```python
from build123d import *

# Parameters (mm, degrees)
SKETCH9_OUTSIDE_W          = 164.226
SKETCH9_OUTSIDE_H          = 164.226
BODY_CUT_DEPTH             = 177.452945975
SKETCH10_OUTSIDE_W         = 127.798
SKETCH10_OUTSIDE_H         = 127.798
BODY_CUT_INNER_DEPTH       = 76.981920155
CUT_FIXING_HOLE_START      = -39.50904
SKETCH15_R                 = 2.75
CUT_FIXING_HOLE_DEPTH      = 39.50904
SKETCH16_R                 = 1.25
CUT_BACK_FIXING_HOLE_DEPTH = 133.739845789
CUT_CORNER_DEPTH           = 160.654828928
CUT_CORNER_INNER_START     = -76.98192
CUT_CORNER_INNER_DEPTH     = 76.98192
SKETCH18_W                 = 2
SKETCH18_H                 = 50.098076211
COSMETIC_FILLET_INNER_R    = 4.3
COSMETIC_FILLET_R          = 4.3


with BuildPart() as part:
    # Sketch5 → Body-Front (revolve)
    with BuildSketch(Plane(origin=(0, 0, 0), x_dir=(0, 0, -1), z_dir=(1, 0, 0)), mode=Mode.PRIVATE) as body_front_sk:
        Polygon((0, 8.339423789), (0, 7.9375), (38.490960077, 7.9375), (38.490960077, 29.153992315), (39.509039923, 29.153992315), (39.509039923, 58.307984631), (0, 58.307984631), (0, 36.5), (-1.5, 36.5), (-1.5, 8.339423789), align=None)
    revolve(body_front_sk.sketch.rotate(Axis((0, 0, -80.9), (0, 0, 1)), 90), axis=Axis((0, 0, -80.9), (0, 0, 1)))

    # Sketch6 → Body-Middle (revolve)
    with BuildSketch(Plane(origin=(0, 0, 0), x_dir=(0, 0, -1), z_dir=(1, 0, 0)), mode=Mode.PRIVATE) as body_middle_sk:
        Polygon((39.509039923, 29.153992315), (39.509039923, 58.307984631), (116.490960077, 58.307984631), (116.490960077, 29.153992315), (117.509039923, 29.153992315), (117.509039923, 7.9375), (38.490960077, 7.9375), (38.490960077, 29.153992315), align=None)
    revolve(body_middle_sk.sketch.rotate(Axis((0, 0, -80.9), (0, 0, 1)), 90), axis=Axis((0, 0, -80.9), (0, 0, 1)))

    # Sketch7 → Body-Back (revolve)
    with BuildSketch(Plane(origin=(0, 0, 0), x_dir=(0, 0, -1), z_dir=(1, 0, 0)), mode=Mode.PRIVATE) as body_back_sk:
        Polygon((156, 58.307984631), (116.490960077, 58.307984631), (116.490960077, 29.153992315), (117.509039923, 29.153992315), (117.509039923, 2.5), (154.5, 2.5), (154.5, 2.901923789), (156, 2.901923789), align=None)
    revolve(body_back_sk.sketch.rotate(Axis((0, 0, -80.9), (0, 0, 1)), 90), axis=Axis((0, 0, -80.9), (0, 0, 1)))

    # Sketch9 outside → Body-Cut (cut, through all)
    with BuildSketch(Plane.XY):
        Rectangle(SKETCH9_OUTSIDE_W, SKETCH9_OUTSIDE_H)
        with BuildLine():
            Line((-36.956744108, 43), (36.956744108, 43))
            ThreePointArc((36.956744108, 43), (41.22997133, 41.22997133), (43, 36.956744108))
            Line((43, 36.956744108), (43, -36.956744108))
            ThreePointArc((43, -36.956744108), (41.22997133, -41.22997133), (36.956744108, -43))
            Line((36.956744108, -43), (-36.956744108, -43))
            ThreePointArc((-36.956744108, -43), (-41.22997133, -41.22997133), (-43, -36.956744108))
            Line((-43, -36.956744108), (-43, 36.956744108))
            ThreePointArc((-43, 36.956744108), (-41.22997133, 41.22997133), (-36.956744108, 43))
        make_face(mode=Mode.SUBTRACT)
    extrude(amount=-BODY_CUT_DEPTH, mode=Mode.SUBTRACT)

    # Sketch10 outside → Body-Cut-Inner (cut)
    with BuildSketch(Plane.XY.offset(-39.509039923)):
        Rectangle(SKETCH10_OUTSIDE_W, SKETCH10_OUTSIDE_H)
        with BuildLine():
            Line((-42.914, 36.956744108), (-42.914, -36.956744108))
            ThreePointArc((-42.914, -36.956744108), (-41.169160146, -41.169160146), (-36.956744108, -42.914))
            Line((-36.956744108, -42.914), (36.956744108, -42.914))
            ThreePointArc((36.956744108, -42.914), (41.169160146, -41.169160146), (42.914, -36.956744108))
            Line((42.914, -36.956744108), (42.914, 36.956744108))
            ThreePointArc((42.914, 36.956744108), (41.169160146, 41.169160146), (36.956744108, 42.914))
            Line((36.956744108, 42.914), (-36.956744108, 42.914))
            ThreePointArc((-36.956744108, 42.914), (-41.169160146, 41.169160146), (-42.914, 36.956744108))
        make_face(mode=Mode.SUBTRACT)
    extrude(amount=-BODY_CUT_INNER_DEPTH, mode=Mode.SUBTRACT)

    # Sketch15 → Cut-Fixing-Hole (cut)
    with BuildSketch(Plane.XY.offset(CUT_FIXING_HOLE_START)):
        with Locations((34.75, -34.75)):
            Circle(SKETCH15_R)
        with Locations((-34.75, -34.75)):
            Circle(SKETCH15_R)
        with Locations((34.75, 34.75)):
            Circle(SKETCH15_R)
        with Locations((-34.75, 34.75)):
            Circle(SKETCH15_R)
    extrude(amount=CUT_FIXING_HOLE_DEPTH, mode=Mode.SUBTRACT)

    # Sketch16 → Cut-Back-Fixing-Hole (cut, through all)
    with BuildSketch(Plane.XY.offset(-116.490960077)):
        with Locations((-23, 0)):
            Circle(SKETCH16_R)
        with Locations((23, 0)):
            Circle(SKETCH16_R)
    extrude(amount=-CUT_BACK_FIXING_HOLE_DEPTH, mode=Mode.SUBTRACT)

    # Sketch11 → Cut-Corner (cut, through all)
    with BuildSketch(Plane.XY.offset(-8.38)):
        with BuildLine():
            Line((-27.349279927, 43), (-27.349279927, 34.75))
            ThreePointArc((-27.349279927, 34.75), (-29.51690065, 29.51690065), (-34.75, 27.349279927))
            Line((-34.75, 27.349279927), (-43, 27.349279927))
            Line((-43, 27.349279927), (-43, 36.956744108))
            ThreePointArc((-43, 36.956744108), (-41.22997133, 41.22997133), (-36.956744108, 43))
            Line((-36.956744108, 43), (-27.349279927, 43))
        make_face()
        with BuildLine():
            Line((-34.75, -27.349279927), (-43, -27.349279927))
            Line((-43, -27.349279927), (-43, -36.956744108))
            ThreePointArc((-43, -36.956744108), (-41.22997133, -41.22997133), (-36.956744108, -43))
            Line((-36.956744108, -43), (-27.349279927, -43))
            Line((-27.349279927, -43), (-27.349279927, -34.75))
            ThreePointArc((-27.349279927, -34.75), (-29.51690065, -29.51690065), (-34.75, -27.349279927))
        make_face()
        with BuildLine():
            Line((27.349279927, -43), (27.349279927, -34.75))
            ThreePointArc((27.349279927, -34.75), (29.51690065, -29.51690065), (34.75, -27.349279927))
            Line((34.75, -27.349279927), (43, -27.349279927))
            Line((43, -27.349279927), (43, -36.956744108))
            ThreePointArc((43, -36.956744108), (41.22997133, -41.22997133), (36.956744108, -43))
            Line((36.956744108, -43), (27.349279927, -43))
        make_face()
        with BuildLine():
            Line((43, 36.956744108), (43, 27.349279927))
            Line((43, 27.349279927), (34.75, 27.349279927))
            ThreePointArc((34.75, 27.349279927), (29.51690065, 29.51690065), (27.349279927, 34.75))
            Line((27.349279927, 34.75), (27.349279927, 43))
            Line((27.349279927, 43), (36.956744108, 43))
            ThreePointArc((36.956744108, 43), (41.22997133, 41.22997133), (43, 36.956744108))
        make_face()
    extrude(amount=-CUT_CORNER_DEPTH, mode=Mode.SUBTRACT)

    # Sketch13 → Cut-Corner-Inner (cut)
    with BuildSketch(Plane.XY.offset(-39.509039923).offset(CUT_CORNER_INNER_START)):
        with BuildLine():
            Line((-34.75, 27.263279927), (-43, 27.263279927))
            Line((-43, 27.263279927), (-43, 36.956744108))
            ThreePointArc((-43, 36.956744108), (-41.22997133, 41.22997133), (-36.956744108, 43))
            Line((-36.956744108, 43), (-27.263279927, 43))
            Line((-27.263279927, 43), (-27.263279927, 34.75))
            ThreePointArc((-27.263279927, 34.75), (-29.456089467, 29.456089467), (-34.75, 27.263279927))
        make_face()
        with BuildLine():
            Line((-34.75, -27.263279927), (-43, -27.263279927))
            Line((-43, -27.263279927), (-43, -36.956744108))
            ThreePointArc((-43, -36.956744108), (-41.22997133, -41.22997133), (-36.956744108, -43))
            Line((-36.956744108, -43), (-27.263279927, -43))
            Line((-27.263279927, -43), (-27.263279927, -34.75))
            ThreePointArc((-27.263279927, -34.75), (-29.456089467, -29.456089467), (-34.75, -27.263279927))
        make_face()
        with BuildLine():
            Line((27.263279927, -43), (27.263279927, -34.75))
            ThreePointArc((27.263279927, -34.75), (29.456089467, -29.456089467), (34.75, -27.263279927))
            Line((34.75, -27.263279927), (43, -27.263279927))
            Line((43, -27.263279927), (43, -36.956744108))
            ThreePointArc((43, -36.956744108), (41.22997133, -41.22997133), (36.956744108, -43))
            Line((36.956744108, -43), (27.263279927, -43))
        make_face()
        with BuildLine():
            Line((43, 36.956744108), (43, 27.263279927))
            Line((43, 27.263279927), (34.75, 27.263279927))
            ThreePointArc((34.75, 27.263279927), (29.456089467, 29.456089467), (27.263279927, 34.75))
            Line((27.263279927, 34.75), (27.263279927, 43))
            Line((27.263279927, 43), (36.956744108, 43))
            ThreePointArc((36.956744108, 43), (41.22997133, 41.22997133), (43, 36.956744108))
        make_face()
    extrude(amount=CUT_CORNER_INNER_DEPTH, mode=Mode.SUBTRACT)

    # Sketch18 → Body-Cable (revolve)
    with BuildSketch(Plane(origin=(0, 0, 0), x_dir=(0, 0, -1), z_dir=(1, 0, 0))):
        with Locations((135.754519961, -27.950961895)):
            Rectangle(SKETCH18_W, SKETCH18_H)
    revolve(axis=Axis((0, 29.153992315, -136.754519961), (0, -1, 0)))

    # Cosmetic-Fillet-Inner
    cosmetic_fillet_inner_edges = [part.edges().sort_by_distance(p)[0] for p in [
        (-27.263279927, 42.914, -77.999999923),
        (-42.914, 27.263279927, -77.999999923),
        (-27.263279927, -42.914, -77.999999923),
        (-42.914, -27.263279927, -77.999999923),
        (42.914, -27.263279927, -77.999999923),
        (27.263279927, -42.914, -77.999999923),
        (42.914, 27.263279927, -77.999999923),
        (27.263279927, 42.914, -77.999999923),
    ]]
    fillet(cosmetic_fillet_inner_edges, radius=COSMETIC_FILLET_INNER_R)

    # Cosmetic-Fillet
    cosmetic_fillet_edges = [part.edges().sort_by_distance(p)[0] for p in [
        (-27.349279927, 43, -23.944519961),
        (-27.349279927, 43, -136.245480039),
        (-43, 27.349279927, -23.944519961),
        (-43, 27.349279927, -136.245480039),
        (-27.349279927, -43, -23.944519961),
        (-43, -27.349279927, -23.944519961),
        (-43, -27.349279927, -136.245480039),
        (-27.349279927, -43, -136.245480039),
        (43, -27.349279927, -23.944519961),
        (27.349279927, -43, -23.944519961),
        (27.349279927, -43, -136.245480039),
        (43, -27.349279927, -136.245480039),
        (27.349279927, 43, -23.944519961),
        (43, 27.349279927, -23.944519961),
        (43, 27.349279927, -136.245480039),
        (27.349279927, 43, -136.245480039),
    ]]
    fillet(cosmetic_fillet_edges, radius=COSMETIC_FILLET_R)


solid = part.part
```
Input: part model. Units: mm. Frame: model coordinates. A direction names the side the tool comes from. Coordinates: 2 decimals unless noted, no trailing zeros. Write each loop counter-clockwise with the first axis right and the second up, starting at its lowest first coordinate (ties: lowest second). Pieces come first, ordered by that corner, then holes.
1) Set-up query: faces 1 (the cylindrical face through (26.12, -41.71, -24.16)), 2 (the flat face through (-38, -35, -8.38)). Return all of +Z, -Z, +X, -X, +Y, -Y with unobstructed straight access to the full face (end or side cutting, diameter ignored); none if empty.
2) Section B-B on x = -14. Output: boundary loops of the cut face in (y, z).
3) Pin query (flat end, axial travel): pin 1 Ø1.2 at (y, z) = (-37.5, -22.5) entering from -X; pin 2 Ø6 at (x, y) = (-0.5, 2.5) entering from +Z; pin 3 Ø1.2 at (x, z) = (-36.5, -75) entering from +Y. Return the tip coordinate at first contact, or that it passes through.
4) Material intervals for line 1 along Y through (x, z) = (-34.75, -6); line 2 along Y through (x, z) = (0, -155.5); line 3 along Y through (x, z) = (34, -1), sorted ascending.
5) Section D-D on x = -30. Output: boundary loops of the cut face in (y, z).
6) Mould query, pull axis Y, two halves, no side actions, for faces 3 (the cylindrical face through (32.723, -32.891, -4.249)), 4 (the flat face through (37, -27.263, -79)), 5 (the flat face through (0, 42.914, -77)). Classes: pulls with the +Y half, pulls with the -Y half, needs draft (parallel to the pull), parting line crosses it, or undercut.
Check result:
1. face 1: -Z, +X, -Y
1. face 2: -Z, -X, -Y
2. outline: (-43, -156) - (43, -156) - (43, -116.49) - (42.91, -116.49) - (42.91, -39.51) - (43, -39.51) - (43, 0) - (33.71, 0) - (33.71, 1.5) - (-33.71, 1.5) - (-33.71, 0) - (-43, 0) - (-43, -39.51) - (-42.91, -39.51) - (-42.91, -116.49) - (-43, -116.49) - close
3. pin 1: stops at x = -27.35
3. pin 2: stops at z = -117.51
3. pin 3: stops at y = 27.26
4. line 1: y = -43 to -37.5, -32 to 32, 37.5 to 43
4. line 2: y = -43 to -2.9, 2.9 to 43
4. line 3: y = -43 to -37.4, -32.1 to 32.1, 37.4 to 43
5. outline: (-43, -8.38) - (-29.07, -8.38) - (-29.07, -39.51) - (-28.96, -39.51) - (-28.96, -116.49) - (-29.07, -116.49) - (-29.07, -156) - (29.07, -156) - (29.07, -116.49) - (28.96, -116.49) - (28.96, -39.51) - (29.07, -39.51) - (29.07, -8.38) - (43, -8.38) - (43, 0) - (20.79, 0) - (20.79, 1.5) - (-20.79, 1.5) - (-20.79, 0) - (-43, 0) - close
6. face 3: undercut
6. face 4: pulls with the -Y half
6. face 5: pulls with the +Y half
